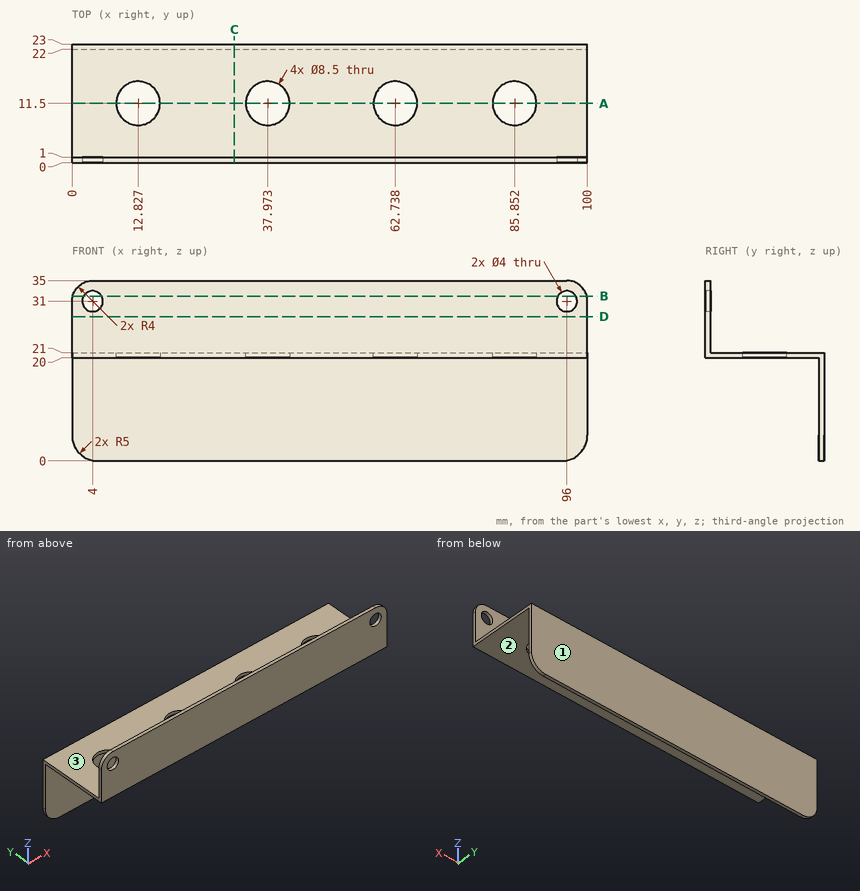
Could you check a few things on this drawing? It's one solid part, dimensions in mm from its lowest x, y, z. A direction names the side the tool comes from. Coordinates: 2 decimals unless noted, no trailing zeros. Write each loop counter-clockwise with the first axis right and the second up, starting at its lowest first coordinate (ties: lowest second). Pieces come first, ordered by that corner, then holes.
Q1. For P1, Ø1, axis at x = 61, y = 18, coming from the +Z side; P2, Ø7, axis at x = 12.83, y = 11.5, coming from the -Z side; P3, Ø6, axis at x = 47.5, y = 11, coming from the -Z side; P4, Ø12, axis at x = 11.5, y = 17, coming from the -Z side, each with a flat end and sliding along its axis, tell me the tip position at first contact or that it passes through.
Results found:
P1: stops at z = 21
P2: passes through
P3: stops at z = 20
P4: stops at z = 0
Q2. Imagine slicing it at B-B, the plane z = 32. List the corners of the cut face in (x, y) for me.
Results found:
outline: (0.13, 0) - (2.27, 0) - (2.27, 1) - (0.13, 1) - close; (5.73, 0) - (94.27, 0) - (94.27, 1) - (5.73, 1) - close; (97.73, 0) - (99.87, 0) - (99.87, 1) - (97.73, 1) - close
Q3. Imagine slicing it at A-A, the plane y = 11.5. List the corners of the cut face in (x, z) for me.
Results found:
outline: (0, 20) - (8.58, 20) - (8.58, 21) - (0, 21) - close; (17.08, 20) - (33.72, 20) - (33.72, 21) - (17.08, 21) - close; (42.22, 20) - (58.49, 20) - (58.49, 21) - (42.22, 21) - close; (66.99, 20) - (81.6, 20) - (81.6, 21) - (66.99, 21) - close; (90.1, 20) - (100, 20) - (100, 21) - (90.1, 21) - close
Q4. Please list where these lines run through material, in increasing order: L1, parallel to X at y = 0.6, z = 31; L2, parallel to Z at x = 4, y = 0.55; L3, parallel to Z at x = 75, y = 2.
Results found:
L1: x = 0 to 2, 6 to 94, 98 to 100
L2: z = 20 to 29, 33 to 35
L3: z = 20 to 21
Q5. Which directions (+Z, -Z, +X, -X, +Y, -Y) give clear straight access to the entire face, cutting with the end or side of a thin tool? Please do the marked faces 1, 2 and 3.
Results found:
face 1: +Z, -Z, +X, -X, +Y
face 2: -Z, +X, -X, -Y
face 3: +Z, +X, -X, +Y
Q6. Imagine slicing it at D-D, the plane z = 28. List the corners of the cut face in (x, y) for me.
Results found:
outline: (0, 0) - (100, 0) - (100, 1) - (0, 1) - close
Q7. Imagine slicing it at C-C, the plane x = 31.5. List the corners of the cut face in (y, z) for me, plus the area to 3 significant figures.
Results found:
outline: (0, 20) - (22, 20) - (22, 0) - (23, 0) - (23, 21) - (1, 21) - (1, 35) - (0, 35) - close
area: 57.0 mm2
